The drawing under review shows one solid part. Ordinate dimensions are in mm from its lowest x, y, z. A direction names the side the tool comes from. Give positions to 0.01 mm unless a question says otherwise; leave off trailing zeros. Order: outer loops, then holes, each group sorted by start corner. A loop starts at its lowest first (then second) coordinate and runs counter-clockwise, first axis right, second up. Notation, with made-up numbers: (74, 49) - (111, 49) arc R32 ccw to (111, 84) - close; hole circle Ø2 at (-17.75, 33.5). An arc over 180 degrees is marked (long way). Use CSV: the item, a comma, the result in double quotes.
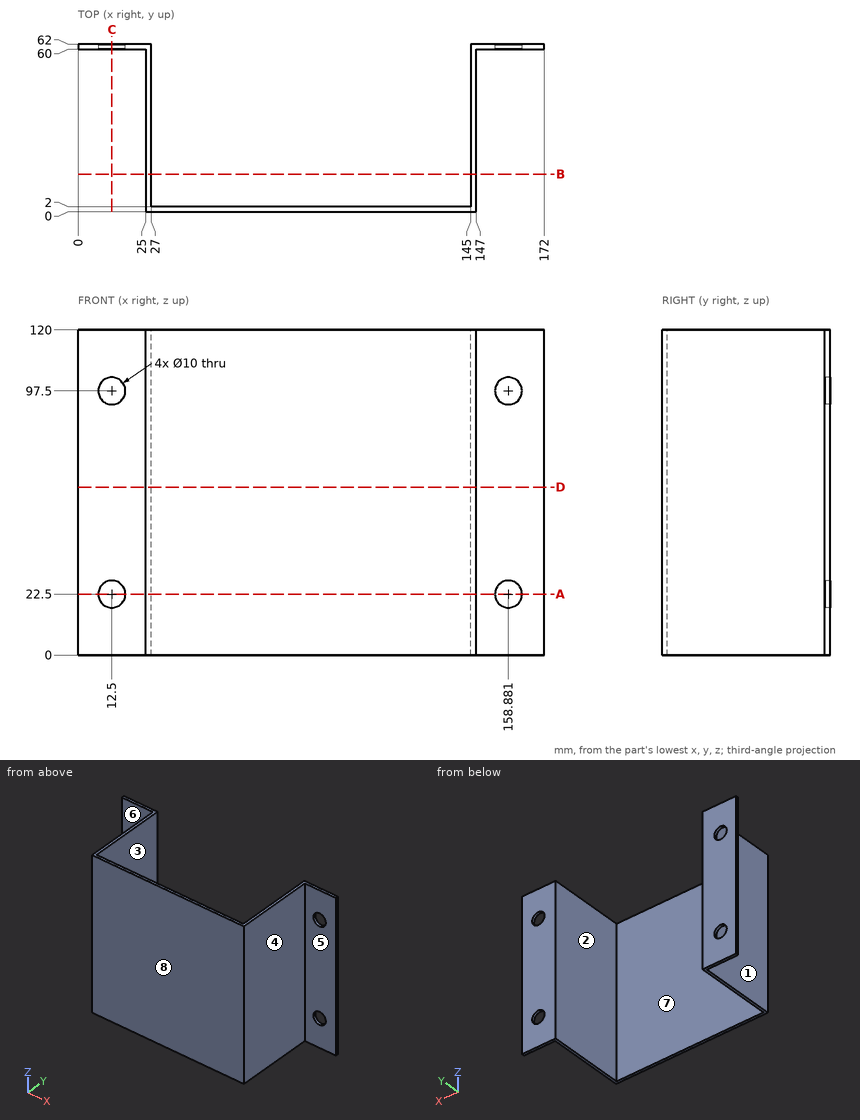
Item 1: Take a section at D-D, the plane z = 62. Give the boundary of the cut face in (x, y).
Results list:
outline,"(0, 60) - (25, 60) - (25, 0) - (147, 0) - (147, 60) - (172, 60) - (172, 62) - (145, 62) - (145, 2) - (27, 2) - (27, 62) - (0, 62) - close"
Item 2: Clearance check with flat-ended pins moving along their axes: pin 1 (18 mm diameter, centred on y = 27, z = 88, fed in from +X); pin 2 (9 mm diameter, centred on x = 158.88, z = 97.5, fed in from -Y); pin 3 (7.5 mm diameter, centred on x = 15.5, z = 63.5, fed in from -Y). State where each tip first meets the part, or that it passes through.
Results list:
pin 1,"stops at x = 147"
pin 2,"passes through"
pin 3,"stops at y = 60"
Item 3: Take a section at B-B, the plane y = 14. Give the boundary of the cut face in (x, z), and give its area (3 significant figures).
Results list:
outline,"(25, 0) - (27, 0) - (27, 120) - (25, 120) - close; (145, 0) - (147, 0) - (147, 120) - (145, 120) - close"
area,"480 mm2"
Item 4: Wall thickness on L1, parallel to Z at x = 12.5, y = 60.7; L2, parallel to X at y = 41.5, z = 36; L3, parallel to Y at x = 158.5, z = 39: over which ranges is each line inside the solid? List them lowest first.
Results list:
L1,"z = 0 to 17.5, 27.5 to 92.5, 102.5 to 120"
L2,"x = 25 to 27, 145 to 147"
L3,"y = 60 to 62"
Item 5: Take a section at C-C, the plane x = 12.5. Give the boundary of the cut face in (y, z).
Results list:
outline,"(60, 0) - (62, 0) - (62, 17.5) - (60, 17.5) - close; (60, 27.5) - (62, 27.5) - (62, 92.5) - (60, 92.5) - close; (60, 102.5) - (62, 102.5) - (62, 120) - (60, 120) - close"
Item 6: Take a section at A-A, the plane z = 22.5. Give the boundary of the cut face in (x, y), and give its area (3 significant figures).
Results list:
outline,"(0, 60) - (7.5, 60) - (7.5, 62) - (0, 62) - close; (17.5, 60) - (25, 60) - (25, 0) - (147, 0) - (147, 60) - (153.88, 60) - (153.88, 62) - (145, 62) - (145, 2) - (27, 2) - (27, 62) - (17.5, 62) - close; (163.88, 60) - (172, 60) - (172, 62) - (163.88, 62) - close"
area,"544 mm2"
Item 7: Tool access review of the marked faces 5, 6, 7 and 8: name each direction out of +Z, -Z, +X, -X, +Y, -Y from which nothing blocks a thin tool from reaching the whole face with its end or side.
Results list:
face 5,"+Z, -Z, +X, -Y"
face 6,"+Z, -Z, -X, -Y"
face 7,"+Z, -Z, +Y"
face 8,"+Z, -Z, +X, -X, -Y"
Item 8: Mouldability with a two-part tool opening along X and no side actions: class the marked faces 1, 2, 3 and 4 as pulls with the +X half, pulls with the -X half, needs draft (parallel to the pull), parting line crosses it, or undercut.
Results list:
face 1,"pulls with the -X half"
face 2,"undercut"
face 3,"undercut"
face 4,"pulls with the +X half"
